Part model, mm, in its own coordinate system. Face numbers are marked on the shaded views. A direction names the side the tool comes from. Round coordinates to 2 decimals unless told otherwise and drop trailing zeros. Order: outer loops, then holes, each group sorted by start corner. A loop starts at its lowest first (then second) coordinate and runs counter-clockwise, first axis right, second up. Notation, with made-up numbers: (84.25, 80.25) - (95.25, 80.25) arc R25 cw to (95.25, 112.25) - close; hole circle Ø9 at (17, 66). An arc over 180 degrees is marked (long way). Return JSON: item names as keys, results as strings. Group by question number.
Item 1: Saw through at B-B on y = -3.5. State how many separate pieces and enclosed holes the cut face has, and give its area (3 significant figures).
Item 2: Probe probe 1 along Z at (x, y) = (17, 5.5); probe 2 along X at (y, z) = (5.75, 36.5); probe 3 along Z at (x, y) = (29, -1). List the from-to ranges inside material, lowest first.
Item 3: Drop flat-ended pins along their axis: pin 1 (1.5 mm diameter, centred on x = 4, z = 64, fed in from -Y); pin 2 (1.1 mm diameter, centred on x = 15, z = 65, fed in from +Y); pin 3 (0.6 mm diameter, centred on x = 30.5, y = 0.5, fed in from -Z). Give the stop position or say it passes through.
Item 4: Saw through at C-C on z = 51.5. List the corners of the cut face in (x, y), and give its area (3 significant figures).
Item 5: Saw through at D-D on x = 19. List the corners of the cut face in (y, z).
Item 6: Two-plate mould, pull along Z, no slides. Class the marked faces 5, 6 and 7: released by +Z, released by -Z, zero draft, split by the parting line, or undercut.
Item 7: Saw through at A-A on x = 29. List the corners of the cut face in (y, z).
Item 8: Tool access for the marked faces 1, 2, 3 and 4: list every direction of +Z, -Z, +X, -X, +Y, -Y with a clear straight run to the whole face (end or side of a thin tool).
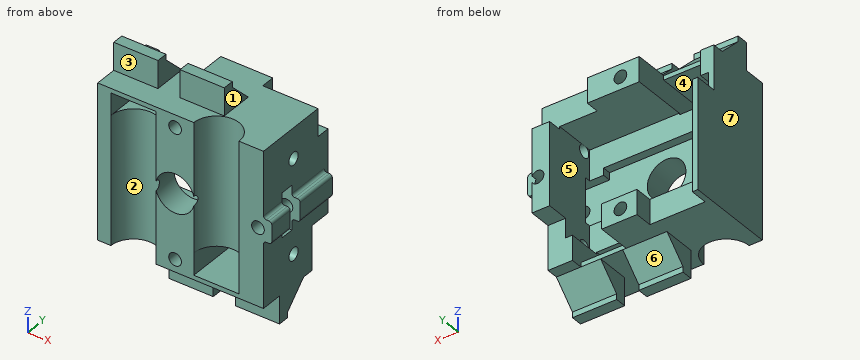
```python
from build123d import *

# Parameters (mm, degrees)
SKETCH1_W           = 28
SKETCH1_H           = 16.1
BOSS_EXTRUDE1_DEPTH = 30
SKETCH2_W           = 10
SKETCH2_H           = 2.5
CUT_EXTRUDE1_DEPTH  = 5
SKETCH3_W           = 10
SKETCH3_H           = 4
CUT_EXTRUDE2_DEPTH  = 8
SKETCH4_W           = 10
SKETCH4_H           = 3.2
CUT_EXTRUDE3_DEPTH  = 8
SKETCH5_W           = 11
SKETCH5_H           = 4
CUT_EXTRUDE4_DEPTH  = 8
SKETCH6_W           = 20
SKETCH6_H           = 2
BOSS_EXTRUDE2_DEPTH = 5
CHAMFER1_SIZE       = 4
SKETCH7_W           = 20
SKETCH7_H           = 2
BOSS_EXTRUDE3_DEPTH = 5
CHAMFER2_SIZE       = 4
SKETCH9_W           = 25.8
SKETCH9_H           = 19
CUT_EXTRUDE6_DEPTH  = 10
SKETCH13_R          = 4.1
CUT_EXTRUDE10_DEPTH = 27.2
SKETCH14_R          = 4.1
CUT_EXTRUDE11_DEPTH = 27.2
SKETCH15_W          = 8.2
SKETCH15_H          = 4
CUT_EXTRUDE12_DEPTH = 27.2
SKETCH16_W          = 0.59230819
SKETCH16_H          = 0.8
SKETCH16_W_2        = 1.617695922
CUT_EXTRUDE13_DEPTH = 4
SKETCH17_W          = 1.5
SKETCH17_H          = 4
BOSS_EXTRUDE4_DEPTH = 16.1
FILLET1_R           = 0.5
SKETCH18_R          = 3.5
CUT_EXTRUDE14_DEPTH = 6.1
SKETCH19_W          = 8
SKETCH19_H          = 1
CUT_EXTRUDE15_DEPTH = 10
SKETCH20_W          = 20.5
SKETCH20_H          = 10.6
CUT_EXTRUDE16_DEPTH = 1.5
SKETCH21_W          = 5.7
SKETCH21_H          = 8
CUT_EXTRUDE17_DEPTH = 1.5
SKETCH22_W          = 8
SKETCH22_H          = 2.5
CUT_EXTRUDE18_DEPTH = 1.5
SKETCH23_R          = 1.15
CUT_EXTRUDE19_DEPTH = 75.620049118
SKETCH24_W          = 8.2
SKETCH24_H          = 0.8
CUT_EXTRUDE20_DEPTH = 2.1
CUT_EXTRUDE21_REACH = 75.421
SKETCH25_W          = 7.929527271
SKETCH25_H          = 1
CUT_EXTRUDE22_START = -5
SKETCH26_W          = 4
SKETCH26_H          = 6
CUT_EXTRUDE22_DEPTH = 5
CUT_EXTRUDE23_START = -5
SKETCH27_W          = 4
SKETCH27_H          = 6
CUT_EXTRUDE23_DEPTH = 5
SKETCH28_R          = 1.15
CUT_EXTRUDE24_DEPTH = 3.2


with BuildPart() as part:
    # Sketch1 → Boss-Extrude1 (new body)
    with BuildSketch(Plane(origin=(0, 0, 0), x_dir=(0, 0, -1), z_dir=(1, 0, 0))):
        with Locations((-46.701535197, -0.990821865)):
            Rectangle(SKETCH1_W, SKETCH1_H)
    extrude(amount=BOSS_EXTRUDE1_DEPTH)

    # Sketch2 → Cut-Extrude1 (cut)
    with BuildSketch(Plane.XY.offset(60.701535197)):
        with Locations((25, 5.809178135)):
            Rectangle(SKETCH2_W, SKETCH2_H)
    extrude(amount=-CUT_EXTRUDE1_DEPTH, mode=Mode.SUBTRACT)

    # Sketch3 → Cut-Extrude2 (cut)
    with BuildSketch(Plane.XY.offset(60.701535197)):
        with Locations((5, 5.059178135)):
            Rectangle(SKETCH3_W, SKETCH3_H)
    extrude(amount=-CUT_EXTRUDE2_DEPTH, mode=Mode.SUBTRACT)

    # Sketch4 → Cut-Extrude3 (cut)
    with BuildSketch(Plane(origin=(0, 0, 32.701535197), x_dir=(-1, 0, 0), z_dir=(0, 0, -1))):
        with Locations((-6, 5.459178135)):
            Rectangle(SKETCH4_W, SKETCH4_H)
    extrude(amount=-CUT_EXTRUDE3_DEPTH, mode=Mode.SUBTRACT)

    # Sketch5 → Cut-Extrude4 (cut)
    with BuildSketch(Plane(origin=(0, 0, 32.701535197), x_dir=(-1, 0, 0), z_dir=(0, 0, -1))):
        with Locations((-24.5, 5.059178135)):
            Rectangle(SKETCH5_W, SKETCH5_H)
    extrude(amount=-CUT_EXTRUDE4_DEPTH, mode=Mode.SUBTRACT)

    # Sketch6 → Boss-Extrude2 (add)
    with BuildSketch(Plane(origin=(0, 0, 32.701535197), x_dir=(-1, 0, 0), z_dir=(0, 0, -1))):
        with Locations((-20, -4.040821865)):
            Rectangle(SKETCH6_W, SKETCH6_H)
    extrude(amount=BOSS_EXTRUDE2_DEPTH)

    # Chamfer1
    chamfer1_edges = [part.edges().sort_by_distance(p)[0] for p in [
        (20, -3.040821865, 32.701535197),
    ]]
    chamfer(chamfer1_edges, length=CHAMFER1_SIZE)

    # Sketch7 → Boss-Extrude3 (add)
    with BuildSketch(Plane.XY.offset(60.701535197)):
        with Locations((10, -4.040821865)):
            Rectangle(SKETCH7_W, SKETCH7_H)
    extrude(amount=BOSS_EXTRUDE3_DEPTH)

    # Chamfer2
    chamfer2_edges = [part.edges().sort_by_distance(p)[0] for p in [
        (10, -3.040821865, 60.701535197),
    ]]
    chamfer(chamfer2_edges, length=CHAMFER2_SIZE)

    # Sketch9 → Cut-Extrude6 (cut)
    with BuildSketch(Plane(origin=(0, 7.059178135, 0), x_dir=(1, 0, 0), z_dir=(0, 1, 0))):
        with Locations((13.9, -46.701535197)):
            Rectangle(SKETCH9_W, SKETCH9_H)
    extrude(amount=-CUT_EXTRUDE6_DEPTH, mode=Mode.SUBTRACT)

    # Sketch13 → Cut-Extrude10 (cut)
    with BuildSketch(Plane.XY.offset(60.701535197)):
        with Locations((21.482304078, -9.040821865)):
            Circle(SKETCH13_R)
    extrude(amount=-CUT_EXTRUDE10_DEPTH, mode=Mode.SUBTRACT)

    # Sketch14 → Cut-Extrude11 (cut)
    with BuildSketch(Plane(origin=(0, 0, 32.701535197), x_dir=(-1, 0, 0), z_dir=(0, 0, -1))):
        with Locations((-6.49230819, -9.040821865)):
            Circle(SKETCH14_R)
    extrude(amount=-CUT_EXTRUDE11_DEPTH, mode=Mode.SUBTRACT)

    # Sketch15 → Cut-Extrude12 (cut)
    with BuildSketch(Plane.XZ.offset(9.040821865)):
        with Locations((6.49230819, 57.901535197)):
            Rectangle(SKETCH15_W, SKETCH15_H)
        with Locations((21.482304078, 35.501535197)):
            Rectangle(SKETCH15_W, SKETCH15_H)
    extrude(amount=-CUT_EXTRUDE12_DEPTH, mode=Mode.SUBTRACT)

    # Sketch16 → Cut-Extrude13 (cut)
    with BuildSketch(Plane(origin=(0, 7.059178135, 0), x_dir=(1, 0, 0), z_dir=(0, 1, 0))):
        with Locations((10.296154095, -60.301535197)):
            Rectangle(SKETCH16_W, SKETCH16_H)
        with Locations((18.191152039, -33.101535197)):
            Rectangle(SKETCH16_W_2, SKETCH16_H)
    extrude(amount=-CUT_EXTRUDE13_DEPTH, mode=Mode.SUBTRACT)

    # Sketch17 → Boss-Extrude4 (add)
    with BuildSketch(Plane.XZ.offset(9.040821865)):
        with Locations((30.75, 46.701535197)):
            Rectangle(SKETCH17_W, SKETCH17_H)
    extrude(amount=-BOSS_EXTRUDE4_DEPTH)

    # Fillet1
    fillet1_edges = [part.edges().sort_by_distance(p)[0] for p in [
        (30, -0.990821865, 44.701535197),
        (30, -0.990821865, 48.701535197),
        (31.5, -0.990821865, 48.701535197),
        (31.5, -0.990821865, 44.701535197),
    ]]
    fillet(fillet1_edges, radius=FILLET1_R)

    # Sketch18 → Cut-Extrude14 (cut)
    with BuildSketch(Plane.XZ.offset(9.040821865)):
        with Locations(Location((13.985, 46.701535197, 0), (0, 0, 194.224464848))):
            Circle(SKETCH18_R)
    extrude(amount=-CUT_EXTRUDE14_DEPTH, mode=Mode.SUBTRACT)

    # Sketch19 → Cut-Extrude15 (cut)
    with BuildSketch(Plane(origin=(31.5, 0, 0), x_dir=(0, 0, -1), z_dir=(1, 0, 0))):
        with Locations((-46.701535197, -2.440821865)):
            Rectangle(SKETCH19_W, SKETCH19_H)
    extrude(amount=-CUT_EXTRUDE15_DEPTH, mode=Mode.SUBTRACT)

    # Sketch20 → Cut-Extrude16 (cut)
    with BuildSketch(Plane(origin=(0, -2.940821865, 0), x_dir=(1, 0, 0), z_dir=(0, 1, 0))):
        with Locations((14.05, -46.701535197)):
            Rectangle(SKETCH20_W, SKETCH20_H)
    extrude(amount=-CUT_EXTRUDE16_DEPTH, mode=Mode.SUBTRACT)

    # Sketch21 → Cut-Extrude17 (cut)
    with BuildSketch(Plane(origin=(0, -2.940821865, 0), x_dir=(1, 0, 0), z_dir=(0, 1, 0))):
        with Locations((27.15, -46.701535197)):
            Rectangle(SKETCH21_W, SKETCH21_H)
    extrude(amount=-CUT_EXTRUDE17_DEPTH, mode=Mode.SUBTRACT)

    # Sketch22 → Cut-Extrude18 (cut)
    with BuildSketch(Plane(origin=(31.5, 0, 0), x_dir=(0, 0, -1), z_dir=(1, 0, 0))):
        with Locations((-46.701535197, -3.190821865)):
            Rectangle(SKETCH22_W, SKETCH22_H)
    extrude(amount=-CUT_EXTRUDE18_DEPTH, mode=Mode.SUBTRACT)

    # Sketch23 → Cut-Extrude19 (cut, through all)
    with BuildSketch(Plane(origin=(0, 7.059178135, 0), x_dir=(1, 0, 0), z_dir=(0, 1, 0))):
        with Locations(Location((29, -46.701535197, 0), (0, 0, 270))):
            Circle(SKETCH23_R)
        with Locations(Location((14, -34.951535197, 0), (0, 0, 270))):
            Circle(SKETCH23_R)
        with Locations(Location((14, -58.451535197, 0), (0, 0, 270))):
            Circle(SKETCH23_R)
    extrude(amount=-CUT_EXTRUDE19_DEPTH, mode=Mode.SUBTRACT)

    # Sketch24 → Cut-Extrude20 (cut)
    with BuildSketch(Plane(origin=(0, 3.059178135, 0), x_dir=(1, 0, 0), z_dir=(0, 1, 0))):
        with Locations((21.482304078, -33.101535197)):
            Rectangle(SKETCH24_W, SKETCH24_H)
        with Locations((6.49230819, -60.301535197)):
            Rectangle(SKETCH24_W, SKETCH24_H)
    extrude(amount=-CUT_EXTRUDE20_DEPTH, mode=Mode.SUBTRACT)

    # Cut-Extrude21: up to this face of the body (flat: up to its plane)
    cut_extrude21_end = Plane(part.part.faces().sort_by_distance((30, -1.445232759, 54.822020691))[0])
    # Sketch25 → Cut-Extrude21 (cut, up to the picked face)
    with BuildSketch(Plane(origin=(31.5, 0, 0), x_dir=(0, 0, -1), z_dir=(1, 0, 0)), mode=Mode.PRIVATE) as cut_extrude21_sk1:
        with Locations((-46.553400254, 6.559178135)):
            Rectangle(SKETCH25_W, SKETCH25_H)
    cut_extrude21_tool1 = split(extrude(cut_extrude21_sk1.sketch, amount=-CUT_EXTRUDE21_REACH, mode=Mode.PRIVATE), bisect_by=cut_extrude21_end, keep=Keep.BOTH, mode=Mode.PRIVATE)
    add(cut_extrude21_tool1.solids().sort_by(Axis((31.5, 6.559178, 46.5534), (-1, 0, 0)))[0], mode=Mode.SUBTRACT)

    # Sketch26 → Cut-Extrude22 (cut)
    with BuildSketch(Plane.XY.offset(65.701535197).offset(CUT_EXTRUDE22_START)):
        with Locations((10, -2.040821865)):
            Rectangle(SKETCH26_W, SKETCH26_H)
    extrude(amount=CUT_EXTRUDE22_DEPTH, mode=Mode.SUBTRACT)

    # Sketch27 → Cut-Extrude23 (cut)
    with BuildSketch(Plane(origin=(0, 0, 27.701535197), x_dir=(-1, 0, 0), z_dir=(0, 0, -1)).offset(CUT_EXTRUDE23_START)):
        with Locations((-20, -2.040821865)):
            Rectangle(SKETCH27_W, SKETCH27_H)
    extrude(amount=CUT_EXTRUDE23_DEPTH, mode=Mode.SUBTRACT)

    # Sketch28 → Cut-Extrude24 (cut)
    with BuildSketch(Plane(origin=(30, 0, 0), x_dir=(0, 0, -1), z_dir=(1, 0, 0))):
        with Locations((-55.201535197, -1.540821865)):
            Circle(SKETCH28_R)
        with Locations((-38.201535197, -1.540821865)):
            Circle(SKETCH28_R)
    extrude(amount=-CUT_EXTRUDE24_DEPTH, mode=Mode.SUBTRACT)


solid = part.part
```
Filled in:
{
 "1": {"separate pieces": "1", "enclosed holes": "4", "area": "663 mm^2"},
 "2": {"probe 1": "z = 32.7 to 37.2, 56.2 to 60.7", "probe 2": "x = 0 to 1, 11 to 17.38", "probe 3": "z = 30.74 to 37.19, 39.22 to 45.55, 47.85 to 54.19, 56.22 to 60.7"},
 "3": {"pin 1": "stops at y = -5.04", "pin 2": "stops at y = -2.79", "pin 3": "stops at z = 44.6"},
 "4": {"outline": "(0, -9.04) - (2.39, -9.04) arc R4.1 cw to (10.59, -9.04) - (17.38, -9.04) arc R4.1 cw to (25.58, -9.04) - (30, -9.04) - (30, 7.06) - (26.8, 7.06) - (26.8, -2.94) - (24.3, -2.94) - (24.3, -4.44) - (3.8, -4.44) - (3.8, -2.94) - (1, -2.94) - (1, 7.06) - (0, 7.06) - close", "area": "141 mm^2"},
 "5": {"outline": "(-9.04, 32.7) - (0.96, 32.7) - (0.96, 33.5) - (-9.04, 33.5) - close; (-5.78, 37.5) - (-2.94, 37.5) - (-2.94, 41.4) - (-4.44, 41.4) - (-4.44, 52) - (-2.94, 52) - (-2.94, 56.2) - (7.06, 56.2) - (7.06, 60.7) - (0.96, 60.7) - (-3.04, 64.7) - (-3.04, 65.7) - (-5.04, 65.7) - (-5.04, 60.7) - (-5.78, 60.7) - close"},
 "6": {"face 5": "undercut", "face 6": "released by -Z", "face 7": "zero draft"},
 "7": {"outline": "(-9.04, 32.7) - (-5.04, 32.7) - (-5.04, 27.7) - (-3.04, 27.7) - (-3.04, 28.7) - (0.96, 32.7) - (3.06, 32.7) - (3.06, 40.7) - (7.06, 40.7) - (7.06, 45.55) - (-1.94, 45.55) - (-1.94, 42.7) - (-4.44, 42.7) - (-4.44, 45.55) - (-9.04, 45.55) - close; (-9.04, 47.85) - (-4.44, 47.85) - (-4.44, 50.7) - (-1.94, 50.7) - (-1.94, 47.85) - (7.06, 47.85) - (7.06, 55.7) - (4.56, 55.7) - (4.56, 60.7) - (-9.04, 60.7) - close; hole circle Ø2.3 at (-1.54, 38.2); hole circle Ø2.3 at (-1.54, 55.2)"},
 "8": {"face 1": "+Z, +X, +Y, -Y", "face 2": "-Z, -Y", "face 3": "+Z, +X, -X, -Y", "face 4": "+Y, -Y"}
}
